Geometry: final body of the model. Coordinates: model frame, mm. A direction names the side the tool comes from. Give positions to 0.01 mm unless a question says otherwise; leave off trailing zeros. Order: outer loops, then holes, each group sorted by start corner. A loop starts at its lowest first (then second) coordinate and runs counter-clockwise, first axis right, second up. Notation, with made-up numbers: (31.5, -9.75) -> (89.5, -9.75) arc R14 ccw to (89.5, 11.25) -> close; hole circle Ø3 at (34, 10.5). An arc over 180 degrees is marked (long way). Answer in a Markdown table with one row per item. Add a question column.
Q1. Line query: line 1 along Z through (x, y) = (-130, -12); line 2 along X through (y, z) = (-10.75, 9); line 3 along X through (y, z) = (0.5, 1). Output: solid intervals per line, ascending. Write a range as from..to.
Q2. Cut plane C-C on x = -89. Return the cut outline in (y, z), and give its area (3 significant figures).
Q3. Contact query for flat-ended pins moving along their axis: P1, Ø5.5, axis at x = -128, z = 7, coming from the -Y side; P2, Ø2, axis at y = 142.5, z = 5, coming from the -X side; P3, Ø13, axis at x = 62.76, y = 172.43, coming from the -Z side; P4, Ø8, axis at x = -59.5, z = 3.5, coming from the +Y side. Output: stop coordinate, or through.
Q4. Set-up query: faces 4 (the face through (-125.6, -8, 9.1)), 5 (the face through (2, 53, 18)). Return all of +Z, -Z, +X, -X, +Y, -Y with unobstructed straight access to the full face (end or side cutting, diameter ignored); none if empty.
Q5. Cut plane A-A on y = 0. Return the cut outline in (x, z).
Q6. Cut plane B-B on y = 95.5. Return the cut outline in (x, z), and give its area (3 significant figures).
Q7. Pull-direction query (X, two-part tool) for faces 1 (the face through (67.585, 186.637, 8.874)), 2 (the face through (-126.034, 11.648, 8.479)), 3 (the face through (2, 53, 0)); classes: +X half, -X half, draft (parallel to the pull), parting line (faces both ways), or undercut.
from build123d import *

# Parameters (mm, degrees)
EXTRUDE_1_DEPTH     = 18
SKETCH_3_R          = 10
SKETCH_3_R_2        = 4
CUT_EXTRUDE_1_DEPTH = 18
SKETCH_4_R          = 4
CUT_EXTRUDE_2_DEPTH = 20
CUT_EXTRUDE_START   = 12
SKETCH_5_W          = 18
SKETCH_5_H          = 16
CUT_EXTRUDE_3_DEPTH = 28
CUT_EXTRUDE_5_DEPTH = 18


with BuildPart() as part:
    # 草图1 → 凸台-拉伸1 (new body)
    with BuildSketch(Plane.XY):
        with BuildLine():
            Line((76.990642, 167.689269), (18.973261, -6.325769))
            ThreePointArc((18.973261, -6.325769), (11.378738, -16.447623), (-0.770942, -19.985136))
            Line((-0.770942, -19.985136), (-130.000001, -15.000028))
            ThreePointArc((-130.000001, -15.000028), (-144.997254, -0.288514), (-130.576922, 14.988929))
            Line((-130.576922, 14.988929), (-23.583521, 19.107084))
            ThreePointArc((-23.583521, 19.107084), (-15.488001, 21.857162), (-10.210075, 28.583518))
            Line((-10.210075, 28.583518), (48.810331, 177.946064))
            ThreePointArc((48.810331, 177.946064), (67.890998, 186.528985), (76.990642, 167.689269))
        make_face()
    extrude(amount=EXTRUDE_1_DEPTH)

    # 草图3 → 切除-拉伸1 (cut)
    with BuildSketch(Plane.XY):
        Circle(SKETCH_3_R)
        with Locations((62.760696, 172.433596)):
            Circle(SKETCH_3_R_2)
    extrude(amount=CUT_EXTRUDE_1_DEPTH, mode=Mode.SUBTRACT)

    # 草图4 → 切除-拉伸2 (cut, symmetric)
    with BuildSketch(Plane(origin=(0, 0, 0), x_dir=(1, 0, 0), z_dir=(0, 1, 0))):
        with Locations(Location((-130, -9, 0), (0, 0, 269.999985))):
            Circle(SKETCH_4_R)
    extrude(amount=CUT_EXTRUDE_2_DEPTH, both=True, mode=Mode.SUBTRACT)

    # 草图5 → 切除-拉伸3 (cut)
    with BuildSketch(Plane(origin=(-130, 0, 0), x_dir=(0, 0, -1), z_dir=(1, 0, 0)).offset(CUT_EXTRUDE_START)):
        with Locations((-9, 0)):
            Rectangle(SKETCH_5_W, SKETCH_5_H)
    extrude(amount=-CUT_EXTRUDE_3_DEPTH, mode=Mode.SUBTRACT)

    # 草图8 → 切除-拉伸5 (cut)
    with BuildSketch(Plane.XY):
        Polygon((-145.000001, 0), (-145.000001, 20), (-138.000001, 20), (-138.000001, -20), (-145.000001, -20), align=None)
    extrude(amount=CUT_EXTRUDE_5_DEPTH, mode=Mode.SUBTRACT)


solid = part.part
Completed:
| question | item | result |
|---|---|---|
| 1 | line 1 | z = 0..5, 13..18 |
| 1 | line 2 | x = -138..-134, -126..16.87 |
| 1 | line 3 | x = -118..-9.99, 9.99..21.25 |
| 2 | outline | (-16.58, 0) -> (16.59, 0) -> (16.59, 18) -> (-16.58, 18) -> close |
| 2 | area | 597 mm² |
| 3 | P1 | stops at y = -15.18 |
| 3 | P2 | stops at x = 34.41 |
| 3 | P3 | stops at z = 0 |
| 3 | P4 | stops at y = 17.88 |
| 4 | face 4 | +Z, -Z, -X |
| 4 | face 5 | +Z, +X, -X, +Y, -Y |
| 5 | outline | (-118, 0) -> (-10, 0) -> (-10, 18) -> (-118, 18) -> close; (10, 0) -> (21.08, 0) -> (21.08, 18) -> (10, 18) -> close |
| 6 | outline | (16.23, 0) -> (52.92, 0) -> (52.92, 18) -> (16.23, 18) -> close |
| 6 | area | 660 mm² |
| 7 | face 1 | parting line |
| 7 | face 2 | undercut |
| 7 | face 3 | draft |
